For this review, take the finished solid that the model builds, in its own axes (mm). A direction names the side the tool comes from. Round coordinates to 2 decimals unless told otherwise and drop trailing zeros. Write each loop counter-clockwise with the first axis right and the second up, starting at its lowest first coordinate (ties: lowest second). Pieces come first, ordered by that corner, then holes. Notation, with made-up numbers: M -3.75,44.5 L 37.25,44.5 A12 ccw 37.25,50.5 Z; hole C 34,41.25 d8. An arc over 180 degrees is marked long. Use one line per item in the form item = value. Start each with the question number.
Item 1: Draft analysis for pull direction Z (two halves, no side actions). For faces 1 (the flat face through (1.3, 2, -0.5)), 2 (the cylindrical face through (4.482, 1.352, 8.674)), 3 (the cylindrical face through (-4.336, -19.524, 0.296)), 4 (the flat face through (1, -3, 10.2)), state which applies: released by +Z, released by -Z, zero draft, split by the parting line, or undercut.
Item 2: For line 1 (Z direction, x = -13, y = 15); line 2 (X direction, y = 0, z = 5); line 3 (Z direction, x = 5, y = 0), list the stretches that pass through material, from the lowest coordinate up. Write a range as [from, to].
Item 3: For faces 5 (the cylindrical face through (2.86, -0.9, -0.25)), 6 (the flat face through (1.3, -2, 10.8)), 7 (the flat face through (0, -9, 4.2)), list the 3-axis set-ups (+Z, -Z, +X, -X, +Y, -Y) from which the entire face can be reached by the end or side of a thin tool; tool diameter is ignored.
Item 4: Add section B-B (z = 8.5). State the section outline as (x, y) points.
Item 5: For P1, Ø3, axis at x = -8.5, y = -13, coming from the -Z side; P2, Ø4.5, axis at y = 0, z = 7.2, coming from the +X side; P3, Ø5, axis at y = 0, z = 7.2, coming from the -X side, all flat-tipped, find the tip position at first contact; note any pin that passes through.
from build123d import *

# Parameters (mm, degrees)
ESQUISSE1_R                  = 20
ESQUISSE1_R_2                = 2.1
BOSS_EXTRU_1_DEPTH           = 4.2
ESQUISSE2_R                  = 7
ESQUISSE2_R_2                = 2.1
BOSS_EXTRU_2_DEPTH           = 6
ESQUISSE3_R                  = 1.5
ENL_V_MAT_EXTRU_1_DEPTH      = 31.067257939
ENL_V_MAT_EXTRU_1_DEPTH_BACK = 31.067257939
ESQUISSE5_R                  = 2
ESQUISSE7_R                  = 3
ESQUISSE7_R_2                = 2.1
BOSS_EXTRU_4_DEPTH           = 0.6
BOSS_EXTRU_5_START           = 0.5
ESQUISSE8_R                  = 3
ESQUISSE8_R_2                = 2.1
BOSS_EXTRU_5_DEPTH           = 0.5


with BuildPart() as part:
    # Esquisse1 → Boss.-Extru.1 (new body)
    with BuildSketch(Plane.XY):
        Circle(ESQUISSE1_R)
        Circle(ESQUISSE1_R_2, mode=Mode.SUBTRACT)
    extrude(amount=BOSS_EXTRU_1_DEPTH)

    # Esquisse2 → Boss.-Extru.2 (add)
    with BuildSketch(Plane.XY.offset(4.2)):
        Circle(ESQUISSE2_R)
        Circle(ESQUISSE2_R_2, mode=Mode.SUBTRACT)
    extrude(amount=BOSS_EXTRU_2_DEPTH)

    # Esquisse3 → Enlèvement de matière-Révolution1 (revolve, cut)
    with BuildSketch(Plane(origin=(0, 0, 0), x_dir=(0, 0, -1), z_dir=(1, 0, 0)), mode=Mode.PRIVATE) as enl_vement_de_mati_re_r_volution1_sk:
        with Locations((-2.1, 20)):
            Circle(ESQUISSE3_R)
    revolve(enl_vement_de_mati_re_r_volution1_sk.sketch.rotate(Axis((0, 0, 0), (0, 0, 1)), 90), axis=Axis((0, 0, 0), (0, 0, 1)), mode=Mode.SUBTRACT)

    # Esquisse5 → Enlèv. mat.-Extru.1 (cut, two sides: drawn at the far end of the back side and taken through both)
    with BuildSketch(Plane(origin=(0, 0, 0), x_dir=(0, 0, -1), z_dir=(1, 0, 0)).offset(-ENL_V_MAT_EXTRU_1_DEPTH_BACK)):
        with Locations((-7.2, 0)):
            Circle(ESQUISSE5_R)
    extrude(amount=ENL_V_MAT_EXTRU_1_DEPTH + ENL_V_MAT_EXTRU_1_DEPTH_BACK, mode=Mode.SUBTRACT)

    # Esquisse7 → Boss.-Extru.4 (add)
    with BuildSketch(Plane.XY.offset(10.2)):
        Circle(ESQUISSE7_R)
        Circle(ESQUISSE7_R_2, mode=Mode.SUBTRACT)
    extrude(amount=BOSS_EXTRU_4_DEPTH)

    # Esquisse8 → Boss.-Extru.5 (add)
    with BuildSketch(Plane(origin=(0, 0, 0), x_dir=(-1, 0, 0), z_dir=(0, 0, -1)).offset(BOSS_EXTRU_5_START)):
        with Locations(Location((0, 0, 0), (0, 0, 180))):
            Circle(ESQUISSE8_R)
        Circle(ESQUISSE8_R_2, mode=Mode.SUBTRACT)
    extrude(amount=-BOSS_EXTRU_5_DEPTH)


solid = part.part
Calculated:
q1.face_1 = released by -Z
q1.face_2 = undercut
q1.face_3 = zero draft
q1.face_4 = released by +Z
q2.line_1 = [0, 0.61], [3.59, 4.2]
q2.line_2 = [-7, -2.1], [2.1, 7]
q2.line_3 = [0, 5.2], [9.2, 10.2]
q3.face_5 = -Z
q3.face_6 = +Z, +X, -X, +Y, -Y
q3.face_7 = +Z
q4.outline = M -6.83,-1.52 A7 ccw 6.83,-1.52 L 1.45,-1.52 A2.1 cw -1.45,-1.52 Z; M -6.83,1.52 L -1.45,1.52 A2.1 cw 1.45,1.52 L 6.83,1.52 A7 ccw Z
q5.P1 = 0
q5.P2 = 7
q5.P3 = -7
